from build123d import *

# Parameters (mm, degrees)
SKETCH1_R           = 12.5
BOSS_EXTRUDE1_DEPTH = 103.5
SKETCH3_R           = 5.101020514
CUT_EXTRUDE1_DEPTH  = 2.8
SKETCH4_R           = 4.25
CUT_EXTRUDE2_DEPTH  = 9.5


with BuildPart() as part:
    # Sketch1 → Boss-Extrude1 (new body)
    with BuildSketch(Plane(origin=(0, 0, 0), x_dir=(1, 0, 0), z_dir=(0, 1, 0))):
        Circle(SKETCH1_R)
    extrude(amount=BOSS_EXTRUDE1_DEPTH)

    # Sketch2 → Cut-Revolve4 (revolve, cut)
    with BuildSketch(Plane(origin=(0, 0, 0), x_dir=(0, 0, -1), z_dir=(1, 0, 0))):
        Polygon((-7.601020514, 103.5), (-12.5, 98.5), (-12.5, 103.5), align=None)
    revolve(axis=Axis((0, 0, 0), (0, 1, 0)), mode=Mode.SUBTRACT)

    # Sketch3 → Cut-Extrude1 (cut)
    with BuildSketch(Plane(origin=(0, 103.5, 0), x_dir=(1, 0, 0), z_dir=(0, 1, 0))):
        Circle(SKETCH3_R)
    extrude(amount=-CUT_EXTRUDE1_DEPTH, mode=Mode.SUBTRACT)

    # Sketch4 → Cut-Extrude2 (cut)
    with BuildSketch(Plane.XZ):
        Circle(SKETCH4_R)
    extrude(amount=-CUT_EXTRUDE2_DEPTH, mode=Mode.SUBTRACT)


solid = part.part
Geometry: final body of the model. Coordinates: model frame, mm. A direction names the side the tool comes from. Coordinates: 2 decimals unless noted, no trailing zeros. Order: outer loops, then holes, each group sorted by start corner. A loop starts at its lowest first (then second) coordinate and runs counter-clockwise, first axis right, second up. Notation, with made-up numbers: (38, 52.5) - (84, 52.5) arc R32 cw to (84, 81.5) - close; hole circle Ø11 at (35, 81). An arc over 180 degrees is marked (long way). Use one line per item in the form item = value.
1) Section A-A (z = 0). Return loops of the section in (x, y).
Solutions:
outline = (-12.5, 0) - (-4.25, 0) - (-4.25, 9.5) - (4.25, 9.5) - (4.25, 0) - (12.5, 0) - (12.5, 98.5) - (7.6, 103.5) - (5.1, 103.5) - (5.1, 100.7) - (-5.1, 100.7) - (-5.1, 103.5) - (-7.6, 103.5) - (-12.5, 98.5) - close
2) Set-up query: faces 5 (the face through (0, 100.7, 0)), 6 (the face through (2.285, 4.684, 3.584)), 7 (the face through (2, 103.5, 5)). Return all of +Z, -Z, +X, -X, +Y, -Y with unobstructed straight access to the full face (end or side cutting, diameter ignored); none if empty.
Solutions:
face_5 = +Y
face_6 = -Y
face_7 = +Z, -Z, +X, -X, +Y
3) Section B-B (y = 56). Return loops of the section in (x, z), then the cut area to 3 significant figures.
Solutions:
outline = circle Ø25 at (0, 0)
area = 491 mm^2
4) Pin query (flat end, axial travel): pin 1 (1.5 mm diameter, centred on y = 76.5, z = 7, fed in from -X); pin 2 (7 mm diameter, centred on x = 0, z = 0, fed in from -Y); pin 3 (1.5 mm diameter, centred on x = -8.5, y = 33, fed in from +Z). Return the tip coordinate at first contact, or that it passes through.
Solutions:
pin_1 = -10.83
pin_2 = 9.5
pin_3 = 9.81
5) Ray query, L1, parallel to Y at x = 2.25, z = -3.75; L2, parallel to Z at x = 0, y = 4.75; L3, parallel to Z at x = 0, y = 101.35. Return the intervals inside material, ascending.
Solutions:
L1 = 0 to 100.7
L2 = -12.5 to -4.25, 4.25 to 12.5
L3 = -9.71 to -5.1, 5.1 to 9.71
6) Mould query, pull axis Z, two halves, no side actions, for faces 1 (the face through (11.547, 48.56, 4.788)), 2 (the face through (0, 0, 5)), 3 (the face through (-0.66, 102.12, -5.06)), 4 (the face through (0, 9.5, 0)). Classes: +Z half, -Z half, draft (parallel to the pull), parting line (faces both ways), or undercut.
Solutions:
face_1 = parting line
face_2 = draft
face_3 = undercut
face_4 = undercut
